Solid Edge part; units mm, degrees
sketch "Sketch1" plane through (0, 0, 0) normal (0, 0, 1) x (1, 0, 0)
  line L0 (0, 9.2) -> (0, 8.575)
  line L1 (0, 8.575) -> (0.15, 8.575)
  arc A0 (0.15, 8.575) -> (0.45, 8.275) centre (0.15, 8.275) cw
  line L2 (0.45, 8.275) -> (0.45, 7.975)
  line L3 (0.45, 7.975) -> (1.5557, 7.975)
  arc A1 (1.5557, 7.975) -> (3.4443, 7.975) centre (2.5, 7.25) cw
  line L4 (3.4443, 7.975) -> (4.55, 7.975)
  line L5 (4.55, 7.975) -> (4.55, 8.275)
  arc A2 (4.55, 8.275) -> (4.85, 8.575) centre (4.85, 8.275) cw
  line L6 (4.85, 8.575) -> (5, 8.575)
  line L7 (5, 8.575) -> (5, 9.2)
  arc A3 (5, 9.2) -> (4.7, 9.5) centre (4.7, 9.2) ccw
  line L8 (4.7, 9.5) -> (0.3, 9.5)
  arc A4 (0.3, 9.5) -> (0, 9.2) centre (0.3, 9.2) ccw
revolve "RevolvedProtrusion1" add sketch "Sketch1" angle 360 about axis through (50, 0, 0) along (-1, 0, 0)
properties part number "SKF_61800-2RS1_or"
Could you check a few things on this model? Use its own coordinates, in mm. Coordinates: 2 decimals unless noted, no trailing zeros. Loops run counter-clockwise (first coordinate to the right, second up) from the corner with the lowest first, then second, coordinate; pieces in that order, holes last.
1) Imagine slicing it at C-C (x = 4.2). List the corners of the cut face in (y, z) for me (3 decimals), and give its area (3 significant figures).
Reported:
outline: circle Ø19 at (0, 0); hole circle Ø15.95 at (0, 0)
area: 83.7 mm2
2) Imagine slicing it at D-D (x = 2.45). List the corners of the cut face in (y, z) for me.
Reported:
outline: circle Ø19 at (0, 0); hole circle Ø16.88 at (0, 0)
3) Will these pins go through, and if not, where does the flat tip stop? pin 1 Ø2 at (x, z) = (4, -3) entering from +Y; pin 2 Ø1.5 at (x, y) = (2.5, 2.5) entering from +Z; pin 3 Ø1.5 at (x, y) = (4.5, -6.5) entering from -Z; pin 4 Ø1 at (y, z) = (6.5, 5.5) entering from +X.
Reported:
pin 1: stops at y = 9.29
pin 2: stops at z = 9.34
pin 3: stops at z = -7.56
pin 4: stops at x = 5
4) Thinking about a two-plate mould opening in Y: for faces 1 (the face through (5, -8, -4)), 2 (the face through (4.005, 7.607, 2.395)), 3 (the face through (2.47, 4.38, 8.43)), 4 (the face through (1.011, 7.607, 2.395)), which applies, released by +Y, released by -Y, zero draft, split by the parting line, or undercut?
Reported:
face 1: zero draft
face 2: undercut
face 3: split by the parting line
face 4: undercut
5) Please list where these lines run through material, in increasing order: line 1 along Y through (x, z) = (4, 0) (3 decimals); line 2 along Z through (x, y) = (3, 4.5).
Reported:
line 1: y = -9.5 to -7.975, 7.975 to 9.5
line 2: z = -8.37 to -7.01, 7.01 to 8.37
6) Imagine slicing it at A-A (y = 0). List the corners of the cut face in (x, z) for me (3 decimals).
Reported:
outline: (0, -9.2) arc R0.3 ccw to (0.3, -9.5) - (4.7, -9.5) arc R0.3 ccw to (5, -9.2) - (5, -8.575) - (4.85, -8.575) arc R0.3 cw to (4.55, -8.275) - (4.55, -7.975) - (3.444, -7.975) arc R1.191 cw to (1.556, -7.975) - (0.45, -7.975) - (0.45, -8.275) arc R0.3 cw to (0.15, -8.575) - (0, -8.575) - close; (0, 8.575) - (0.15, 8.575) arc R0.3 cw to (0.45, 8.275) - (0.45, 7.975) - (1.556, 7.975) arc R1.191 cw to (3.444, 7.975) - (4.55, 7.975) - (4.55, 8.275) arc R0.3 cw to (4.85, 8.575) - (5, 8.575) - (5, 9.2) arc R0.3 ccw to (4.7, 9.5) - (0.3, 9.5) arc R0.3 ccw to (0, 9.2) - close
